Verification items for this drawing (mm, ordinates from the low corner). A direction names the side the tool comes from. Coordinates: 2 decimals unless noted, no trailing zeros. Write each loop counter-clockwise with the first axis right and the second up, starting at its lowest first coordinate (ties: lowest second). Pieces come first, ordered by that corner, then holes. Notation, with made-up numbers: (31, 65) -> (63, 65) arc R21 cw to (63, 104) -> close; hole circle Ø8 at (-4, -7). An arc over 180 degrees is marked (long way). Use CSV: the item, a comma, the result in double quotes.
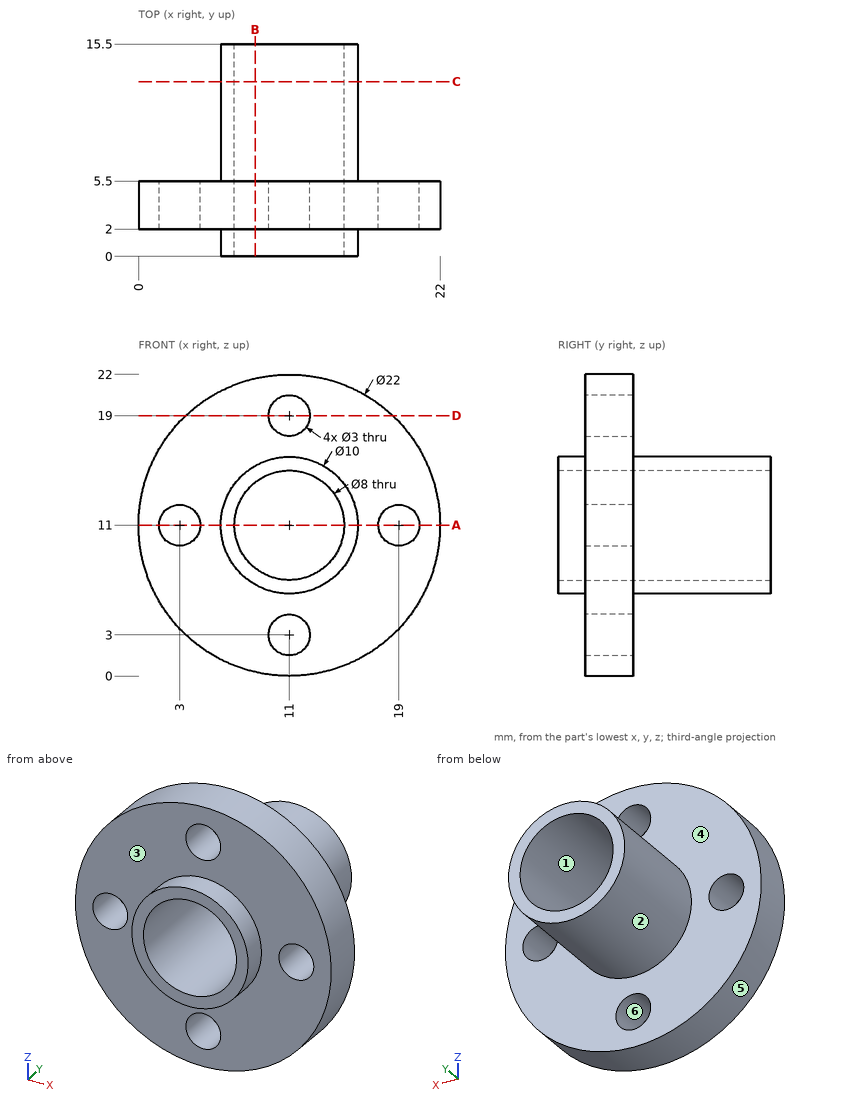
1) Cross-section at C-C (y = 12.75). Record the boundary of the cut face in (x, z).
Return value:
outline,"circle Ø10 at (11, 11); hole circle Ø8 at (11, 11)"
2) Set-up check for the marked faces 1, 2 and 3: record each of +Z, -Z, +X, -X, +Y, -Y from which the full face is reachable in a straight line by a thin tool's end or side.
Return value:
face 1,"+Y, -Y"
face 2,"+Y"
face 3,"-Y"
3) Cross-section at D-D (z = 19). Record the boundary of the cut face in (x, y), plus the area to 3 significant figures.
Return value:
outline,"(3.45, 2) -> (9.5, 2) -> (9.5, 5.5) -> (3.45, 5.5) -> close; (12.5, 2) -> (18.55, 2) -> (18.55, 5.5) -> (12.5, 5.5) -> close"
area,"42.3 mm2"
4) Cross-section at A-A (z = 11). Record the boundary of the cut face in (x, y), plus the area to 3 significant figures.
Return value:
outline,"(0, 2) -> (1.5, 2) -> (1.5, 5.5) -> (0, 5.5) -> close; (4.5, 2) -> (6, 2) -> (6, 0) -> (7, 0) -> (7, 15.5) -> (6, 15.5) -> (6, 5.5) -> (4.5, 5.5) -> close; (15, 0) -> (16, 0) -> (16, 2) -> (17.5, 2) -> (17.5, 5.5) -> (16, 5.5) -> (16, 15.5) -> (15, 15.5) -> close; (20.5, 2) -> (22, 2) -> (22, 5.5) -> (20.5, 5.5) -> close"
area,"52.0 mm2"
5) Mould release check, pull along X, two halves, no side actions. Record for the marked faces 4, 5 and 6: released by +X, released by -X, zero draft, split by the parting line, or undercut.
Return value:
face 4,"zero draft"
face 5,"split by the parting line"
face 6,"undercut"
6) Cross-section at B-B (x = 8.5). Record the boundary of the cut face in (y, z), plus the area to 3 significant figures.
Return value:
outline,"(0, 6.67) -> (2, 6.67) -> (2, 0.29) -> (5.5, 0.29) -> (5.5, 6.67) -> (15.5, 6.67) -> (15.5, 7.88) -> (0, 7.88) -> close; (0, 14.12) -> (15.5, 14.12) -> (15.5, 15.33) -> (5.5, 15.33) -> (5.5, 21.71) -> (2, 21.71) -> (2, 15.33) -> (0, 15.33) -> close"
area,"82.1 mm2"
7) Scan lines: L1, parallel to X at y = 3.4, z = 11; L2, parallel to Y at x = 11, z = 5; L3, parallel to X at y = 9.75, z = 12.25. Record each from-to range of solid material in increasing order.
Return value:
L1,"0 to 1.5, 4.5 to 7, 15 to 17.5, 20.5 to 22"
L2,"2 to 5.5"
L3,"6.16 to 7.2, 14.8 to 15.84"
8) Gauge pin test, flat ends, axial feed: pin 1 (2 mm diameter, centred on y = 3, z = 7.5, fed in from +X); pin 2 (3 mm diameter, centred on y = 8.5, z = 5, fed in from -X); pin 3 (4 mm diameter, centred on y = 6.5, z = 5.5, fed in from -X); pin 4 (2.5 mm diameter, centred on x = 19, z = 11, fed in from -Y) (3 decimals). Record the tip position at first contact, or that the pin passes through.
Return value:
pin 1,"x = 21.71"
pin 2,"x = 8.82"
pin 3,"x = 0.67"
pin 4,"through"
